CAD build for the part. Positions are in the model's coordinates, mm. A direction names the side the tool comes from. Coordinates: 2 decimals unless noted, no trailing zeros. Order: outer loops, then holes, each group sorted by start corner. A loop starts at its lowest first (then second) coordinate and runs counter-clockwise, first axis right, second up. Notation, with made-up numbers: (-6.75, -33.75) - (0.25, -33.75) arc R18 cw to (0.25, -24.75) - close; hole circle Ø5 at (-16, -13). An arc over 180 degrees is marked (long way). Return JSON: item names as keys, results as strings.
from build123d import *

# Parameters (mm, degrees)
F0_R     = 30.5
F0_R_2   = 2.555
F0_R_3   = 8.265
F1_DEPTH = 7.94
F2_SIZE  = 0.4
F0_R_4   = 4.765
F3_DEPTH = 9.53
F4_SIZE  = 0.2


with BuildPart() as f1:
    # F0 (on Top) → F1 (new body)
    with BuildSketch(Plane.XY):
        Circle(F0_R)
        with Locations((-18, -18)):
            Circle(F0_R_2, mode=Mode.SUBTRACT)
        with Locations((18, -18)):
            Circle(F0_R_2, mode=Mode.SUBTRACT)
        with BuildLine():
            ThreePointArc((-18, 15.445), (-19.806658, 19.806658), (-15.445, 18))
            ThreePointArc((-15.445, 18), (-16.193342, 16.193342), (-18, 15.445))
        make_face(mode=Mode.SUBTRACT)
        Circle(F0_R_3, mode=Mode.SUBTRACT)
        with Locations((18, 18)):
            Circle(F0_R_2, mode=Mode.SUBTRACT)
    extrude(amount=F1_DEPTH)

    # F2
    f2_edges = [f1.edges().sort_by_distance(p)[0] for p in [
        (-30.5, 0, 7.94),
    ]]
    chamfer(f2_edges, length=F2_SIZE)

    # F0 (on Top) → F3 (join)
    with BuildSketch(Plane.XY):
        Circle(F0_R_3)
        Circle(F0_R_4, mode=Mode.SUBTRACT)
    extrude(amount=F3_DEPTH)

    # F4
    f4_edges = [f1.edges().sort_by_distance(p)[0] for p in [
        (-8.265, 0, 9.53),
    ]]
    chamfer(f4_edges, length=F4_SIZE)


solid = f1.part
Item 1: Drop flat-ended pins along their axis: P1, Ø3, axis at y = 12, z = 8, coming from the -X side; P2, Ø2, axis at y = 12.5, z = 5.5, coming from the -X side; P3, Ø6, axis at x = 18, y = 18, coming from the +Z side; P4, Ø4.5, axis at x = 18, y = -18, coming from the +Z side. Give the stop position or say it passes through.
Findings below:
{"P1": "stops at x = -28.61", "P2": "stops at x = -28.25", "P3": "stops at z = 7.94", "P4": "passes through"}
Item 2: Band-saw the part on C-C, the plane y = -18. Count the separate pieces of the cut face and the enclosed holes in it, then the cut area to 3 significant figures.
Findings below:
{"separate pieces": "3", "enclosed holes": "0", "area": "310 mm²"}
Item 3: Which spindle directions (+Z, -Z, +X, -X, +Y, -Y) get a long thin tool onto all of the face, cutting with end or side? Do faces 4 (the cylindrical face through (-19.88, -16.27, 3.91)), 5 (the flat face through (6, -6, 7.94)). Say none if no direction does.
Findings below:
{"face 4": "+Z, -Z", "face 5": "+Z"}
Item 4: Band-saw the part on A-A, the plane x = 0. List the corners of the cut face in (y, z) (3 decimals), then the cut area to 3 significant figures.
Findings below:
{"outline": "(-30.5, 0) - (-4.765, 0) - (-4.765, 9.53) - (-8.065, 9.53) - (-8.265, 9.33) - (-8.265, 7.94) - (-30.1, 7.94) - (-30.5, 7.54) - close; (4.765, 0) - (30.5, 0) - (30.5, 7.54) - (30.1, 7.94) - (8.265, 7.94) - (8.265, 9.33) - (8.065, 9.53) - (4.765, 9.53) - close", "area": "420 mm²"}
Item 5: Band-saw the part on B-B, the plane z = 2.5. List the corners of the cut face in (x, y) (3 decimals), then the cut area to 3 significant figures.
Findings below:
{"outline": "circle Ø61 at (0, 0); hole circle Ø5.11 at (-18, -18); hole circle Ø5.11 at (-18, 18); hole circle Ø9.53 at (0, 0); hole circle Ø5.11 at (18, -18); hole circle Ø5.11 at (18, 18)", "area": "2,770 mm²"}
Item 6: Wall check: L1, parallel to X at y = 17, z = 1.75; L2, parallel to Y at x = -20, z = 1; L3, parallel to X at y = -17.5, z = 3.75. Give the ranges that are in metal, low to high. Write a range as [from, to].
Findings below:
{"L1": "x = [-25.32, -20.35], [-15.65, 15.65], [20.35, 25.32]", "L2": "y = [-23.03, -19.59], [-16.41, 16.41], [19.59, 23.03]", "L3": "x = [-24.98, -20.51], [-15.49, 15.49], [20.51, 24.98]"}
Item 7: Mould opens along X. For faces 1 (the cylindrical face through (7.883, 2.483, 8.625)), 2 (the flat face through (3.5, -3.5, 9.53)), 3 (the cylindrical face through (16.12, -16.27, 3.91)) say: released by +X, released by -X, zero draft, split by the parting line, or undercut.
Findings below:
{"face 1": "split by the parting line", "face 2": "zero draft", "face 3": "undercut"}
